Can you work these out from the model? Positions are in its coordinate system, mm. Give positions to 0.01 mm unless a question says otherwise; leave off trailing zeros. Write each loop counter-clockwise with the first axis right and the second up, starting at its lowest first coordinate (ties: lowest second). Pieces come first, ordered by that corner, then holes. Notation, with made-up numbers: (11, 16.25) -> (22, 16.25) arc R12 cw to (22, 23.25) -> close; hole circle Ø1 at (65.25, 2.25). An arc over 180 degrees is marked (long way). One line per item, written item: value.
from build123d import *

# Parameters (mm, degrees)
ESQUISSE1_R        = 1.5
ESQUISSE1_R_2      = 2.5
BOSS_EXTRU_1_DEPTH = 2
CONG_1_R           = 12


with BuildPart() as part:
    # Esquisse1 → Boss.-Extru.1 (new, symmetric)
    with BuildSketch(Plane(origin=(0, 29.5, 0), x_dir=(1, 0, 0), z_dir=(0, 1, 0))):
        with BuildLine():
            Line((56.491378029, -49.493903346), (45.612572194, -60.37270918))
            ThreePointArc((45.612572194, -60.37270918), (41.468560381, -68.255453254), (42.524007936, -77.09833279))
            ThreePointArc((42.524007936, -77.09833279), (40.447621803, -84.488468372), (32.803300859, -83.788582233))
            Line((32.803300859, -83.788582233), (28.914213562, -79.899494937))
            ThreePointArc((28.914213562, -79.899494937), (20.428932188, -77.071067812), (17.600505063, -68.585786438))
            Line((17.600505063, -68.585786438), (13.711417767, -64.696699141))
            ThreePointArc((13.711417767, -64.696699141), (13.011531628, -57.052378197), (20.40166721, -54.975992064))
            ThreePointArc((20.40166721, -54.975992064), (29.244546746, -56.031439619), (37.12729082, -51.887427806))
            Line((37.12729082, -51.887427806), (48.006096654, -41.008621971))
            ThreePointArc((48.006096654, -41.008621971), (56.491378029, -41.008621971), (56.491378029, -49.493903346))
        make_face()
        with Locations(Location((17.954058454, -60.454058454, 0), (0, 0, 270))):
            Circle(ESQUISSE1_R, mode=Mode.SUBTRACT)
        with Locations(Location((37.045941546, -79.545941546, 0), (0, 0, 90))):
            Circle(ESQUISSE1_R, mode=Mode.SUBTRACT)
        with Locations(Location((27.5, -70, 0), (0, 0, 270))):
            Circle(ESQUISSE1_R_2, mode=Mode.SUBTRACT)
        with Locations(Location((52.248737342, -45.251262658, 0), (0, 0, 270))):
            Circle(ESQUISSE1_R_2, mode=Mode.SUBTRACT)
    extrude(amount=BOSS_EXTRU_1_DEPTH, both=True)

    # Congé1
    cong_1_edges = [part.edges().sort_by_distance(p)[0] for p in [
        (28.914213562, 29.5, 79.899494937),
        (17.600505063, 29.5, 68.585786438),
    ]]
    fillet(cong_1_edges, radius=CONG_1_R)


solid = part.part
1) If we section it at C-C (y = 29.25): Write out the boundary of the cut face in (x, z).
Answer list:
outline: (13.71, 64.7) arc R6 ccw to (20.4, 54.98) arc R15 cw to (37.13, 51.89) -> (48.01, 41.01) arc R6 ccw to (56.49, 49.49) -> (45.61, 60.37) arc R15 cw to (42.52, 77.1) arc R6 ccw to (32.8, 83.79) -> (32.2, 83.19) arc R12 cw to (25.78, 79.85) arc R10 ccw to (17.65, 71.72) arc R12 cw to (14.31, 65.3) -> close; hole circle Ø3 at (17.95, 60.45); hole circle Ø5 at (27.5, 70); hole circle Ø3 at (37.05, 79.55); hole circle Ø5 at (52.25, 45.25)
2) I need wall thicknesses on L1, parallel to Z at x = 53, y = 28.05; L2, parallel to X at y = 28.9, z = 61; L3, parallel to X at y = 29.4, z = 78.5. Which ranges of each line are inside material? Lowest first, please.
Answer list:
L1: z = 39.3 to 42.87, 47.64 to 52.99
L2: x = 11.98 to 16.56, 19.35 to 45.02
L3: x = 22.23 to 35.97, 38.12 to 42.95
3) If we section it at D-D (z = 75.5): Write out the boundary of the cut face in (x, y).
Answer list:
outline: (19.15, 27.5) -> (41.92, 27.5) -> (41.92, 31.5) -> (19.15, 31.5) -> close
4) We'd pull the mould along Z, two halves only. Please class faces 1 (the face through (41.5, 29.5, 68.1)), 2 (the face through (35, 27.5, 62)), 3 (the face through (30, 29, 70)), 4 (the face through (51.128, 29.528, 54.857)): released by +Z, released by -Z, zero draft, split by the parting line, or undercut.
Answer list:
face 1: undercut
face 2: zero draft
face 3: undercut
face 4: released by +Z
5) If we section it at A-A (z = 68.5): Write out the boundary of the cut face in (x, y), and give its area (3 significant figures).
Answer list:
outline: (16.6, 27.5) -> (25.5, 27.5) -> (25.5, 31.5) -> (16.6, 31.5) -> close; (29.5, 27.5) -> (41.43, 27.5) -> (41.43, 31.5) -> (29.5, 31.5) -> close
area: 83.3 mm^2
6) If we section it at B-B (x = 27.5): Write out the boundary of the cut face in (y, z), and give its area (3 significant figures).
Answer list:
outline: (27.5, 56.25) -> (31.5, 56.25) -> (31.5, 67.5) -> (27.5, 67.5) -> close; (27.5, 72.5) -> (31.5, 72.5) -> (31.5, 80.28) -> (27.5, 80.28) -> close
area: 76.1 mm^2
7) Will these pins go through, and if not, where does the flat tip stop? pin 1 (1 mm diameter, centred on y = 28.5, z = 74.5, fed in from -X); pin 2 (1.5 mm diameter, centred on y = 30.5, z = 49, fed in from +X); pin 3 (1.5 mm diameter, centred on y = 30.5, z = 70, fed in from -X).
Answer list:
pin 1: stops at x = 18.33
pin 2: stops at x = 57.45
pin 3: stops at x = 16.94
